Can you work these out from the model? Positions are in its coordinate system, mm. Face numbers are marked on the shaded views. Coordinates: 2 decimals unless noted, no trailing zeros. Order: outer loops, then holes, each group sorted by start corner. A loop starts at its lowest first (then second) coordinate and runs counter-clockwise, first axis right, second up.
```python
from build123d import *

# Parameters (mm, degrees)
CUT_EXTRUDE1_START = 11.2776
CUT_EXTRUDE1_DEPTH = 1.7526


with BuildPart() as part:
    # Sketch2 → Revolve1 (revolve)
    with BuildSketch(Plane(origin=(0, 0, 0), x_dir=(0, 0, -1), z_dir=(1, 0, 0)), mode=Mode.PRIVATE) as revolve1_sk:
        with BuildLine():
            Line((11.2776, 0), (11.2776, 1.27635))
            Line((11.2776, 1.27635), (10.80135, 1.7526))
            Line((10.80135, 1.7526), (-7.7724, 1.7526))
            Line((-7.7724, 1.7526), (-7.7724, 2.69494))
            ThreePointArc((-7.7724, 2.69494), (-7.823732466, 2.818867534), (-7.94766, 2.8702))
            Line((-7.94766, 2.8702), (-11.10234, 2.8702))
            ThreePointArc((-11.10234, 2.8702), (-11.226267534, 2.818867534), (-11.2776, 2.69494))
            Line((-11.2776, 2.69494), (-11.2776, 0))
            Line((-11.2776, 0), (11.2776, 0))
        make_face()
    revolve(revolve1_sk.sketch.rotate(Axis((0, 0, -11.2776), (0, 0, 1)), 90), axis=Axis((0, 0, -11.2776), (0, 0, 1)))

    # Sketch3 → Cut-Extrude1 (cut)
    with BuildSketch(Plane.XY.offset(CUT_EXTRUDE1_START)):
        Polygon((-1.3890625, 0.801975608), (-1.3890625, -0.801975608), (0, -1.603951217), (1.3890625, -0.801975608), (1.3890625, 0.801975608), (0, 1.603951217), align=None)
    extrude(amount=-CUT_EXTRUDE1_DEPTH, mode=Mode.SUBTRACT)

    # Cut-Extrude2 cone 1 section (through the dimple's axis) → Cut-Extrude2 (revolve, cut)
    with BuildSketch(Plane(origin=(0, 0, 11.2776), x_dir=(0, -1, 0), z_dir=(1, 0, 0))):
        Polygon((0, 0), (1.78578268, 0), (0, 1.031022111), align=None)
    revolve(axis=Axis((0, 0, 11.2776), (0, 0, -1)), mode=Mode.SUBTRACT)


solid = part.part
```
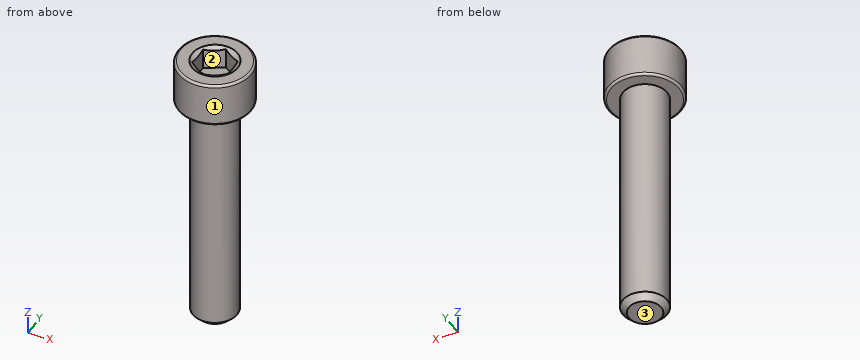
1. I'm going to push flat-ended pins straight in: pin 1 (0.8 mm diameter, centred on x = 0, y = 0, fed in from +Z) (3 decimals); pin 2 (1.5 mm diameter, centred on x = 1, z = -3, fed in from +Y); pin 3 (1 mm diameter, centred on x = 0.5, y = 1, fed in from +Z). Where does each tip first touch, or does it pass through?
Completed:
pin 1: stops at z = 9.525
pin 2: stops at y = 1.73
pin 3: stops at z = 11.18
2. Imagine slicing it at A-A on y = 0. Please give me the cut outline in (x, z) (3 decimals).
Completed:
outline: (-2.87, 7.948) arc R0.175 ccw to (-2.695, 7.772) - (-1.753, 7.772) - (-1.753, -10.801) - (-1.276, -11.278) - (1.276, -11.278) - (1.753, -10.801) - (1.753, 7.772) - (2.695, 7.772) arc R0.175 ccw to (2.87, 7.948) - (2.87, 11.102) arc R0.175 ccw to (2.695, 11.278) - (1.786, 11.278) - (1.389, 11.049) - (1.389, 9.525) - (-1.389, 9.525) - (-1.389, 11.049) - (-1.786, 11.278) - (-2.695, 11.278) arc R0.175 ccw to (-2.87, 11.102) - close
3. Please list where these lines run through material, in increasing order: probe 1 along Z at (x, y) = (0.1, -0.3) (3 decimals); probe 2 along Z at (x, y) = (-2.55, 0.95); probe 3 along Y at (x, z) = (-1, 5.75).
Completed:
probe 1: z = -11.278 to 9.525
probe 2: z = 7.77 to 11.28
probe 3: y = -1.44 to 1.44
4. Imagine slicing it at B-B on z = -0.75. Please give me the cut outline in (x, y).
Completed:
outline: circle Ø3.51 at (0, 0)
5. Thinking about a two-plate mould opening in Y: for the marked faces 1, 2 and 3, which applies, pulls with the +Y half, pulls with the -Y half, needs draft (parallel to the pull), parting line crosses it, or undercut?
Completed:
face 1: parting line crosses it
face 2: undercut
face 3: needs draft
